The figure shows three views and two pictorial views of one solid part (mm, origin at its lowest corner). Answer the questions. A direction names the side the tool comes from. Coordinates: 2 decimals unless noted, no trailing zeros. Write each loop counter-clockwise with the first axis right and the second up, starting at its lowest first coordinate (ties: lowest second). Pieces come first, ordered by that corner, then holes. Notation, with made-up numbers: (31.5, -30) - (53.5, -30) arc R29 ccw to (53.5, 9) - close; hole circle Ø5 at (-5.75, 58.5). An arc over 180 degrees is marked (long way). Use a Markdown table: item, result. Add a question column.
(1) The part is cut by section D-D, the plane x = 30. Give the vertices of the cut face in (y, z).
(2) Given pin 1 Ø6 at (x, z) = (31, 16) entering from +Y; pin 2 Ø3 at (x, z) = (55.5, 5) entering from -Y; pin 3 Ø5 at (y, z) = (173.5, 15) entering from -X, each flat-ended and moving along its own axis, determine where each tip first touches the part or whether it passes through.
(3) A tool of negligible diameter and unlimited length cuts with its end or side. For the marked faces 1 and 2, from which of +Z, -Z, +X, -X, +Y, -Y can it reach the whole face along a straight path? Write none if from no direction.
(4) The part is cut by section A-A, the plane y = 173. Give the vertices of the cut face in (x, z), then the cut area to 3 significant figures.
(5) The part is cut by section B-B, the plane z = 21.5. Give the vertices of the cut face in (x, y).
(6) Find the intervals of material crossed by line 1 (Y direction, x = 86, z = 21.5); line 2 (Z direction, x = 86, y = 173); line 3 (Y direction, x = 85, z = 21), in increasing order. Write a range as from..to.
(7) The part is cut by section C-C, the plane z = 34. Give the vertices of the cut face in (x, y).
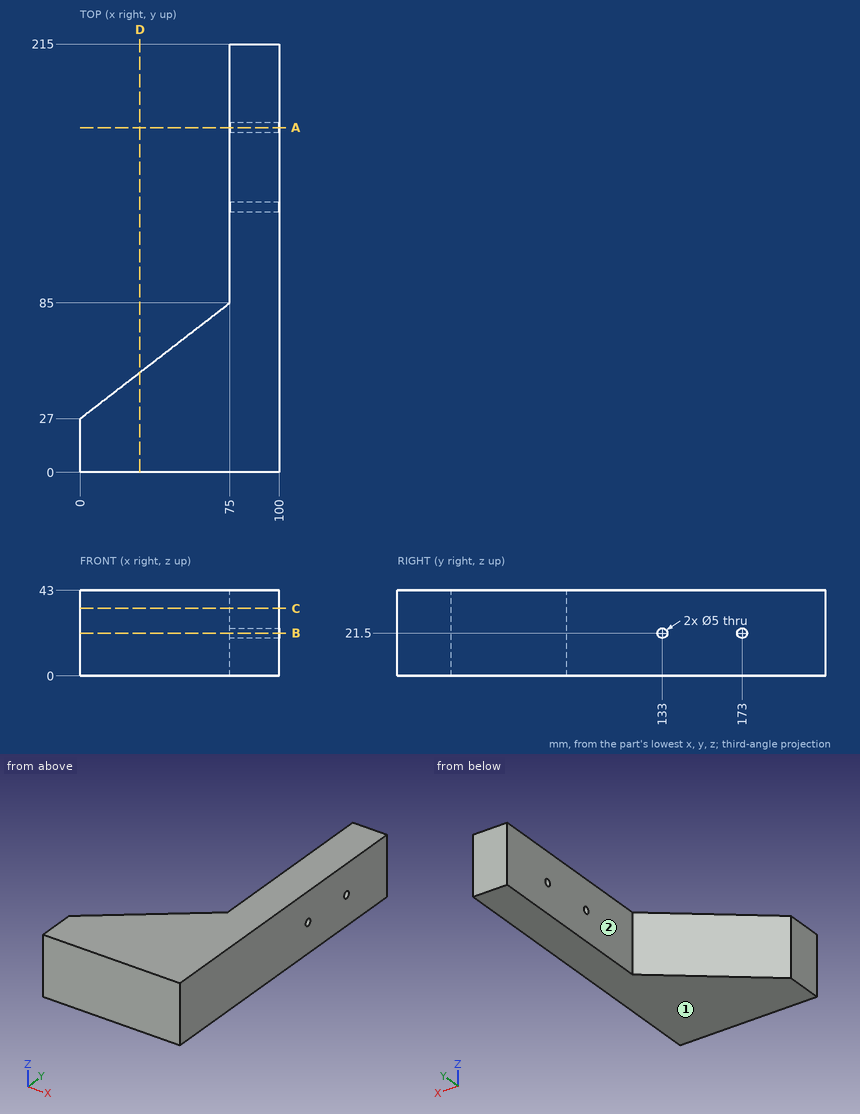
Model answer:
| question | item | result |
|---|---|---|
| 1 | outline | (0, 0) - (50.2, 0) - (50.2, 43) - (0, 43) - close |
| 2 | pin 1 | y = 53.29 |
| 2 | pin 2 | y = 0 |
| 2 | pin 3 | x = 75 |
| 3 | face 1 | -Z, +X, -X, +Y, -Y |
| 3 | face 2 | +Z, -Z, -X, +Y |
| 4 | outline | (75, 0) - (100, 0) - (100, 19) - (75, 19) - close; (75, 24) - (100, 24) - (100, 43) - (75, 43) - close |
| 4 | area | 950 mm^2 |
| 5 | outline | (0, 0) - (100, 0) - (100, 130.5) - (75, 130.5) - (75, 85) - (0, 27) - close; (75, 135.5) - (100, 135.5) - (100, 170.5) - (75, 170.5) - close; (75, 175.5) - (100, 175.5) - (100, 215) - (75, 215) - close |
| 6 | line 1 | 0..130.5, 135.5..170.5, 175.5..215 |
| 6 | line 2 | 0..19, 24..43 |
| 6 | line 3 | 0..130.55, 135.45..170.55, 175.45..215 |
| 7 | outline | (0, 0) - (100, 0) - (100, 215) - (75, 215) - (75, 85) - (0, 27) - close |
